Could you check a few things on this model? Use its own coordinates, in mm. A direction names the side the tool comes from. Coordinates: 2 decimals unless noted, no trailing zeros. Loops run counter-clockwise (first coordinate to the right, second up) from the corner with the lowest first, then second, coordinate; pieces in that order, holes last. Notation, with made-up numbers: M 82,-37 L 129,-37 A30 ccw 129,-11 Z; hole C -13,-16.75 d10. An arc over 180 degrees is marked long. Return JSON: item names as keys, results as strings. Group by question number.
from build123d import *

# Parameters (mm, degrees)
SKETCH1_R           = 6.35
BOSS_EXTRUDE1_DEPTH = 12.7
FILLET1_R           = 6.35


with BuildPart() as part:
    # Sketch1 → Boss-Extrude1 (new body)
    with BuildSketch(Plane.XY):
        with BuildLine():
            Line((-85.102216058, -9.525), (-16.497783942, -9.525))
            ThreePointArc((-16.497783942, -9.525), (19.05, 0), (-16.497783942, 9.525))
            Line((-16.497783942, 9.525), (-85.102216058, 9.525))
            ThreePointArc((-85.102216058, 9.525), (-120.65, 0), (-85.102216058, -9.525))
        make_face()
        Circle(SKETCH1_R, mode=Mode.SUBTRACT)
        with Locations((-101.6, 0)):
            Circle(SKETCH1_R, mode=Mode.SUBTRACT)
    extrude(amount=BOSS_EXTRUDE1_DEPTH)

    # Fillet1
    fillet1_edges = [part.edges().sort_by_distance(p)[0] for p in [
        (-85.102216058, 9.525, 6.35),
        (-16.497783942, 9.525, 6.35),
        (-16.497783942, -9.525, 6.35),
        (-85.102216058, -9.525, 6.35),
    ]]
    fillet(fillet1_edges, radius=FILLET1_R)


solid = part.part
(1) Imagine slicing it at A-A, the plane y = 0. Write out the boundary of the cut face in (x, z), then the cut area to 3 significant figures.
(2) For faces 1 (the face through (-120.64, 0.66, 6.26)), 2 (the face through (-51, -9.525, 6)), 3 (the face through (-50, 9.525, 6)), which set-ups out of +Z, -Z, +X, -X, +Y, -Y let a thin tool reach every point of the face, with its end or its side?
(3) If I drill on L1, parallel to Y at x = 0, z = 7.5; L2, parallel to X at y = 4, z = 2.75; L3, parallel to Y at x = -54.5, z = 5.25 (3 decimals), over which ranges is the centre line in solid material (lowest first)? Write a range as [from, to].
(4) Imagine slicing it at C-C, the plane z = 4.5. Write out the boundary of the cut face in (x, y) (3 decimals).
(5) We'd pull the mould along X, two halves only. Please class faces 4 (the face through (-17.04, 10.17, 6.44)), 5 (the face through (-52, 0, 0)), 6 (the face through (-17.114, -10.134, 6.439)): +X half, -X half, draft (parallel to the pull), parting line (faces both ways), or undercut.
(6) Imagine slicing it at D-D, the plane y = 15. Write out the boundary of the cut face in (x, z).
(7) Imagine slicing it at B-B, the plane x = 0. Write out the boundary of the cut face in (y, z), then the cut area to 3 significant figures.
(8) Will these pins go through, and if not, where does the flat tip stop? P1, Ø3, axis at x = -54, z = 7, coming from the +Y side (3 decimals); P2, Ø3, axis at x = -98.5, z = 3.5, coming from the -Y side; P3, Ø6, axis at x = -13, z = 10, coming from the -Y side; P4, Ø11.5, axis at x = 0, y = 0, coming from the -Z side.
Checks:
{
 "1": {"outline": "M -120.65,0 L -107.95,0 L -107.95,12.7 L -120.65,12.7 Z; M -95.25,0 L -6.35,0 L -6.35,12.7 L -95.25,12.7 Z; M 6.35,0 L 19.05,0 L 19.05,12.7 L 6.35,12.7 Z", "area": "1,450 mm²"},
 "2": {"face 1": "+Z, -Z", "face 2": "+Z, -Z, -Y", "face 3": "+Z, -Z, +Y"},
 "3": {"L1": "[-19.05, -6.35], [6.35, 19.05]", "L2": "[-120.23, -106.53], [-96.67, -4.93], [4.93, 18.63]", "L3": "[-9.525, 9.525]"},
 "4": {"outline": "M -86.729,-11.906 A6.35 cw -81.772,-9.525 L -19.828,-9.525 A6.35 cw -14.871,-11.906 A19.05 ccw long -14.871,11.906 A6.35 cw -19.828,9.525 L -81.772,9.525 A6.35 cw -86.729,11.906 A19.05 ccw long Z; hole C -101.6,0 d12.7; hole C 0,0 d12.7"},
 "5": {"face 4": "undercut", "face 5": "draft", "face 6": "undercut"},
 "6": {"outline": "M -113.34,0 L -89.86,0 L -89.86,12.7 L -113.34,12.7 Z; M -11.74,0 L 11.74,0 L 11.74,12.7 L -11.74,12.7 Z"},
 "7": {"outline": "M -19.05,0 L -6.35,0 L -6.35,12.7 L -19.05,12.7 Z; M 6.35,0 L 19.05,0 L 19.05,12.7 L 6.35,12.7 Z", "area": "323 mm²"},
 "8": {"P1": "y = 9.525", "P2": "y = -18.98", "P3": "y = -16.21", "P4": "through"}
}
